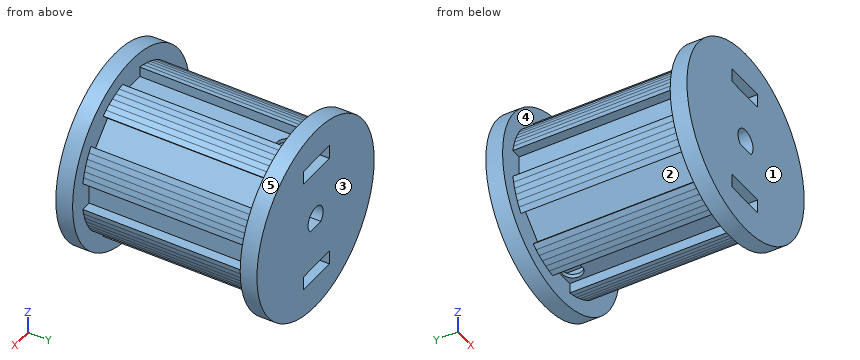
from build123d import *

# Parameters (mm, degrees)
SKETCH1_R           = 17
BOSS_EXTRUDE1_DEPTH = 3
SKETCH3_R           = 17
BOSS_EXTRUDE2_DEPTH = 3
BOSS_EXTRUDE3_DEPTH = 31
SKETCH7_R           = 1.751351815
CUT_EXTRUDE11_DEPTH = 50
CUT_EXTRUDE1_DEPTH  = 50
SKETCH8_W           = 7.5
SKETCH8_H           = 2.5
CUT_EXTRUDE12_DEPTH = 40


with BuildPart() as part:
    # Sketch1 → Boss-Extrude1 (new body)
    with BuildSketch(Plane(origin=(0, -15, 0), x_dir=(1, 0, 0), z_dir=(0, 1, 0))):
        with Locations(Location((0, 0, 0), (0, 0, 270))):
            Circle(SKETCH1_R)
    extrude(amount=BOSS_EXTRUDE1_DEPTH)



with BuildPart() as body_2:
    # Sketch3 → Boss-Extrude2 (new body)
    with BuildSketch(Plane(origin=(0, 21, 0), x_dir=(1, 0, 0), z_dir=(0, 1, 0))):
        with Locations(Location((0, 0, 0), (0, 0, 270))):
            Circle(SKETCH3_R)
    extrude(amount=-BOSS_EXTRUDE2_DEPTH)


with BuildPart() as part_1:
    add(part.part)

    add(body_2.part)  # Boss-Extrude3 merges body 2
    # Sketch6 → Boss-Extrude3 (add)
    with BuildSketch(Plane(origin=(0, -12, 0), x_dir=(1, 0, 0), z_dir=(0, 1, 0))):
        Polygon((-10.39609313, -6.860559341), (-11.68775931, -8.152225055), (-12.244775891, -7.288892753), (-12.738139369, -6.387668662), (-13.165283017, -5.453239195), (-13.523988426, -4.490460269), (-13.812389225, -3.504338907), (-14.028987847, -2.499999944), (-12.202296406, -2.499999944), (-12.202296406, 2.499999944), (-14.028987847, 2.499999944), (-13.812389225, 3.504338907), (-13.523988426, 4.490460269), (-13.165283017, 5.453239195), (-12.738139369, 6.387668662), (-12.244775891, 7.288892753), (-11.68775931, 8.152225055), (-10.39609313, 6.860559341), (-6.860559341, 10.39609313), (-8.152225055, 11.68775931), (-7.288892753, 12.244775891), (-6.387668662, 12.738139369), (-5.453239195, 13.165283017), (-4.490460269, 13.523988426), (-3.504338907, 13.812389225), (-2.499999944, 14.028987847), (-2.499999944, 12.174172863), (2.499999944, 12.202296406), (2.499999944, 14.028987847), (3.504338907, 13.812389225), (4.490460269, 13.523988426), (5.453239195, 13.165283017), (6.387668662, 12.738139369), (7.288892753, 12.244775891), (8.152225055, 11.68775931), (6.860559341, 10.39609313), (10.39609313, 6.860559341), (11.68775931, 8.152225055), (12.244775891, 7.288892753), (12.738139369, 6.387668662), (13.165283017, 5.453239195), (13.523988426, 4.490460269), (13.812389225, 3.504338907), (14.028987847, 2.499999944), (12.202296406, 2.499999944), (12.202296406, -2.499999944), (14.028987847, -2.499999944), (13.812389225, -3.504338907), (13.523988426, -4.490460269), (13.165283017, -5.453239195), (12.738139369, -6.387668662), (12.244775891, -7.288892753), (11.68775931, -8.152225055), (10.39609313, -6.860559341), (6.860559341, -10.39609313), (8.152225055, -11.68775931), (7.288892753, -12.244775891), (6.387668662, -12.738139369), (5.453239195, -13.165283017), (4.490460269, -13.523988426), (3.504338907, -13.812389225), (2.499999944, -14.028987847), (2.499999944, -12.202296406), (-2.499999944, -12.202296406), (-2.499999944, -14.028987847), (-3.504338907, -13.812389225), (-4.490460269, -13.523988426), (-5.453239195, -13.165283017), (-6.387668662, -12.738139369), (-7.288892753, -12.244775891), (-8.152225055, -11.68775931), (-6.860559341, -10.39609313), align=None)
    extrude(amount=BOSS_EXTRUDE3_DEPTH)

    # Sketch7 → Cut-Extrude11 (cut)
    with BuildSketch(Plane(origin=(-0.068553102, 0, -12.187849043), x_dir=(-0.9999841817006155, 0, 0.005624619858302935), z_dir=(-0.005624619858302935, 0, -0.9999841817006155))):
        with Locations((-0.120761258, 16)):
            Circle(SKETCH7_R)
    extrude(amount=-CUT_EXTRUDE11_DEPTH, mode=Mode.SUBTRACT)

    # Sketch2 → Cut-Extrude1 (cut)
    with BuildSketch(Plane(origin=(0, -15, 0), x_dir=(1, 0, 0), z_dir=(0, 1, 0))):
        with BuildLine():
            Line((1.514793699, 1.566442938), (-1.521232282, 1.566442938))
            ThreePointArc((-1.521232282, 1.566442938), (-0.003219291, -2.164389177), (1.514793699, 1.566442938))
        make_face()
    extrude(amount=CUT_EXTRUDE1_DEPTH, mode=Mode.SUBTRACT)

    # Sketch8 → Cut-Extrude12 (cut)
    with BuildSketch(Plane(origin=(0, -15, 0), x_dir=(1, 0, 0), z_dir=(0, 1, 0))):
        with Locations((-0.237061367, 10.255385433)):
            Rectangle(SKETCH8_W, SKETCH8_H)
    cut_extrude12 = extrude(amount=CUT_EXTRUDE12_DEPTH, mode=Mode.SUBTRACT)

    # Mirror1: Cut-Extrude12 across plane
    add(cut_extrude12.mirror(Plane.XY), mode=Mode.SUBTRACT)


solid = part_1.part
Read the model definition and answer for the solid it produces. Units are mm, in the model's axes. Face numbers are marked on the shaded views. A direction names the side the tool comes from. Round coordinates to 2 decimals unless told otherwise and drop trailing zeros. Write each loop counter-clockwise with the first axis right and the second up, starting at its lowest first coordinate (ties: lowest second). Pieces come first, ordered by that corner, then holes.
1. Which of the six approach directions +Z, -Z, +X, -X, +Y, -Y give full straight-line access (tool end or side, diameter ignored) to the marked faces 4 and 5?
2. Straight lines are drawn through the part: L1, parallel to Z at x = -1, y = -5; L2, parallel to Y at x = 14, z = -0.5; L3, parallel to X at y = 5, z = 0. For each, find the intervals that lie inside material, in ascending order.
3. The part is cut by section D-D, the plane z = 0. Determine the outline of the cut face in (x, y).
4. Determine the mould class of the marked faces 1, 2 and 3 for opening direction Y: pulls with the +Y half, pulls with the -Y half, needs draft (parallel to the pull), parting line crosses it, or undercut.
5. The part is cut by section B-B, the plane y = 2. State how many separate pieces and enclosed holes the cut face has, then the cut area to 3 significant figures.
6. The part is cut by section A-A, the plane z = -15. Determine the outline of the cut face in (x, y).
7. Given pin 1 Ø5 at (x, y) = (-12, 5) entering from -Z; pin 2 Ø1.5 at (y, z) = (1, -4.5) entering from +X; pin 3 Ø2 at (x, y) = (0.5, -3) entering from +Z; pin 4 Ø2.5 at (x, z) = (0, -0.01) entering from +Y, each flat-ended and moving along its own axis, determine where each tip first touches the part or whether it passes through.
Values:
1. face 4: none
1. face 5: +Y, -Y
2. L1: z = -12.18 to -11.51, -9.01 to -1.57, 1.92 to 9.01, 11.51 to 12.2
2. L2: y = -15 to -12, 18 to 21
2. L3: x = -12.2 to -2.18, 2.17 to 12.2
3. outline: (-17, -15) - (-2.18, -15) - (-2.18, 21) - (-17, 21) - (-17, 18) - (-12.2, 18) - (-12.2, -12) - (-17, -12) - close; (2.17, -15) - (17, -15) - (17, -12) - (12.2, -12) - (12.2, 18) - (17, 18) - (17, 21) - (2.17, 21) - close
4. face 1: pulls with the -Y half
4. face 2: undercut
4. face 3: pulls with the +Y half
5. separate pieces: 1
5. enclosed holes: 3
5. area: 508 mm2
6. outline: (-8, -15) - (8, -15) - (8, -12) - (-8, -12) - close; (-8, 18) - (8, 18) - (8, 21) - (-8, 21) - close
7. pin 1: stops at z = -8.15
7. pin 2: stops at x = 13.74
7. pin 3: stops at z = 12.2
7. pin 4: passes through
